from build123d import *

# Parameters (mm, degrees)
SKETCH1_R           = 6
SKETCH1_R_2         = 5
BOSS_EXTRUDE1_DEPTH = 10
SKETCH2_R           = 9.5
CUT_EXTRUDE1_DEPTH  = 6
CUT_EXTRUDE3_DEPTH  = 11
FILLET1_R           = 2
M4_TAPPED_HOLE1_D   = 3


with BuildPart() as part:
    # Sketch1 → Boss-Extrude1 (new body)
    with BuildSketch(Plane(origin=(0, 0, 0), x_dir=(1, 0, 0), z_dir=(0, 1, 0))):
        with BuildLine():
            Line((-14.758368201, -9.680542044), (-11.496273776, -137.792727273))
            ThreePointArc((-11.496273776, -137.792727273), (0, -149), (11.496273776, -137.792727273))
            Line((11.496273776, -137.792727273), (14.758368201, -9.680542044))
            ThreePointArc((14.758368201, -9.680542044), (15.433257, -8.135337646), (16.995139708, -7.5))
            Line((16.995139708, -7.5), (16.995139708, 7.5))
            ThreePointArc((16.995139708, 7.5), (13.895638119, 8.122041636), (11.276155185, 9.891831188))
            ThreePointArc((11.276155185, 9.891831188), (0.004561048, 14.999999307), (-11.270137484, 9.898686836))
            ThreePointArc((-11.270137484, 9.898686836), (-13.891539017, 8.123905388), (-16.995139708, 7.5))
            Line((-16.995139708, 7.5), (-16.995139708, -7.5))
            ThreePointArc((-16.995139708, -7.5), (-15.433257, -8.135337646), (-14.758368201, -9.680542044))
        make_face()
        Circle(SKETCH1_R, mode=Mode.SUBTRACT)
        with Locations((0, -137.5)):
            Circle(SKETCH1_R_2, mode=Mode.SUBTRACT)
    extrude(amount=BOSS_EXTRUDE1_DEPTH)

    # Sketch2 → Cut-Extrude1 (cut)
    with BuildSketch(Plane(origin=(0, 10, 0), x_dir=(1, 0, 0), z_dir=(0, 1, 0))):
        with Locations((0, -137.5)):
            Circle(SKETCH2_R)
    extrude(amount=-CUT_EXTRUDE1_DEPTH, mode=Mode.SUBTRACT)

    # Sketch4 → Cut-Extrude3 (cut, through all)
    with BuildSketch(Plane(origin=(0, 0, 0), x_dir=(1, 0, 0), z_dir=(0, 1, 0))):
        with BuildLine():
            Line((-9.376393506, -24.618181818), (-8.443776056, -61.244852893))
            ThreePointArc((-8.443776056, -61.244852893), (0, -69.476363636), (8.443776056, -61.244852893))
            Line((8.443776056, -61.244852893), (9.376393506, -24.618181818))
            ThreePointArc((9.376393506, -24.618181818), (0, -15), (-9.376393506, -24.618181818))
        make_face()
        with BuildLine():
            Line((-7.90050824, -82.580601653), (-6.96789079, -119.207272727))
            ThreePointArc((-6.96789079, -119.207272727), (0, -126), (6.96789079, -119.207272727))
            Line((6.96789079, -119.207272727), (7.90050824, -82.580601653))
            ThreePointArc((7.90050824, -82.580601653), (0, -74.476363636), (-7.90050824, -82.580601653))
        make_face()
    extrude(amount=CUT_EXTRUDE3_DEPTH, mode=Mode.SUBTRACT)

    # Fillet1
    fillet1_edges = [part.edges().sort_by_distance(p)[0] for p in [
        (-16.995139708, 5, 7.5),
        (-16.995139708, 5, -7.5),
        (16.995139708, 5, -7.5),
        (16.995139708, 5, 7.5),
    ]]
    fillet(fillet1_edges, radius=FILLET1_R)

    # M4 Tapped Hole1 (through all)
    with Locations(Plane.ZY.offset(16.995139708)):
        with Locations((0, 5)):
            Hole(M4_TAPPED_HOLE1_D / 2)


solid = part.part
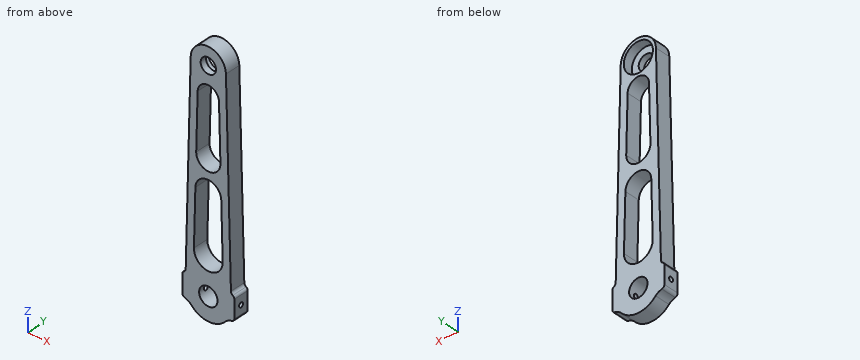
Read the model definition and answer for the solid it produces. Units are mm, in the model's axes. Coordinates: 2 decimals unless noted, no trailing zeros. Loops run counter-clockwise (first coordinate to the right, second up) from the corner with the lowest first, then second, coordinate; pieces in that order, holes last. Notation, with made-up numbers: (15, 71.25) -> (25, 71.25) arc R21 ccw to (25, 79.25) -> close; hole circle Ø11 at (9, 9.25). An arc over 180 degrees is marked (long way). Answer in a Markdown table with one row per item.
Item 1: A cutting plane is placed at B-B on x = 0. Determine the outline of the cut face in (y, z).
Returned:
| item | result |
|---|---|
| outline | (0, -15) -> (10, -15) -> (10, -6) -> (0, -6) -> close; (0, 6) -> (10, 6) -> (10, 15) -> (0, 15) -> close; (0, 69.48) -> (10, 69.48) -> (10, 74.48) -> (0, 74.48) -> close; (0, 126) -> (10, 126) -> (10, 128) -> (4, 128) -> (4, 132.5) -> (0, 132.5) -> close; (0, 142.5) -> (4, 142.5) -> (4, 147) -> (10, 147) -> (10, 149) -> (0, 149) -> close |
Item 2: A cutting plane is placed at C-C on y = 2. Determine the outline of the cut face in (x, z) (1 decimal).
Returned:
| item | result |
|---|---|
| outline | (-17, -5.7) arc R2 ccw to (-15.4, -7.7) arc R8 cw to (-11.3, -9.9) arc R15 ccw to (11.3, -9.9) arc R8 cw to (15.4, -7.7) arc R2 ccw to (17, -5.7) -> (17, 6) arc R2 ccw to (15.9, 7.8) arc R2.2 cw to (14.8, 9.7) -> (11.5, 137.8) arc R11.5 ccw to (-11.5, 137.8) -> (-14.8, 9.7) arc R2.2 cw to (-15.9, 7.8) arc R2 ccw to (-17, 6) -> close; hole (-9.4, 24.6) arc R9.4 ccw (long way) to (9.4, 24.6) -> (8.4, 61.2) arc R8.4 ccw to (-8.4, 61.2) -> close; hole (-7.9, 82.6) arc R7.9 ccw (long way) to (7.9, 82.6) -> (7, 119.2) arc R7 ccw to (-7, 119.2) -> close; hole circle Ø12 at (0, 0); hole circle Ø10 at (0, 137.5) |
Item 3: A cutting plane is placed at A-A on z = 0. Determine the outline of the cut face in (x, y).
Returned:
| item | result |
|---|---|
| outline | (-17, 0) -> (-6, 0) -> (-6, 3.5) -> (-17, 3.5) -> close; (-17, 6.5) -> (-6, 6.5) -> (-6, 10) -> (-17, 10) -> close; (6, 0) -> (17, 0) -> (17, 3.5) -> (6, 3.5) -> close; (6, 6.5) -> (17, 6.5) -> (17, 10) -> (6, 10) -> close |
Item 4: Each of these flat-tipped pins is pushed along its axis until it touches: P1, Ø3, axis at y = 5, z = 34, coming from the -X side; P2, Ø1, axis at x = -7, y = 2.5, coming from the +Z side. Where does it stop, or does it pass through?
Returned:
| item | result |
|---|---|
| P1 | stops at x = -14.18 |
| P2 | stops at z = 146.99 |
Item 5: A cutting plane is placed at D-D on z = 31. Determine the outline of the cut face in (x, y), plus the area to 3 significant figures.
Returned:
| item | result |
|---|---|
| outline | (-14.22, 0) -> (-9.21, 0) -> (-9.21, 10) -> (-14.22, 10) -> close; (9.21, 0) -> (14.22, 0) -> (14.22, 10) -> (9.21, 10) -> close |
| area | 100 mm^2 |
Item 6: Straight lines are drawn through the part: line 1 along Y through (x, z) = (-11.25, 0); line 2 along Z through (x, y) = (-4, 1.5); line 3 along X through (y, z) = (0.85, 137.5). For each, find the intervals that lie inside material, in ascending order. Write a range as [from, to].
Returned:
| item | result |
|---|---|
| line 1 | y = [0, 3.5], [6.5, 10] |
| line 2 | z = [-14.46, -4.47], [4.47, 15.9], [68.47, 75.56], [124.74, 134.5], [140.5, 148.28] |
| line 3 | x = [-11.5, -5], [5, 11.5] |
